from build123d import *

# Parameters (mm, degrees)
CROQUIS1_W              = 36
CROQUIS1_H              = 25
SALIENTE_EXTRUIR1_DEPTH = 25
CROQUIS2_W              = 31
CROQUIS2_H              = 25
CORTAR_EXTRUIR1_DEPTH   = 22
CROQUIS3_R              = 2.15
CORTAR_EXTRUIR2_DEPTH   = 37
CROQUIS3_3_R            = 2.65
CROQUIS3_3_R_2          = 2.15
CORTAR_EXTRUIR3_DEPTH   = 1.015
CROQUIS4_R              = 2.65
CROQUIS4_R_2            = 2.15
CORTAR_EXTRUIR4_DEPTH   = 1.015
CROQUIS5_W              = 31
CROQUIS5_H              = 25
SALIENTE_EXTRUIR2_DEPTH = 22
CROQUIS6_W              = 25.17
CROQUIS6_H              = 25
CORTAR_EXTRUIR5_DEPTH   = 22
CROQUIS8_R              = 2.15
CORTAR_EXTRUIR6_DEPTH   = 34.5
CROQUIS8_3_R            = 2.65
CROQUIS8_3_R_2          = 2.15
CORTAR_EXTRUIR7_DEPTH   = 1.015
CROQUIS10_R             = 2.65
CROQUIS10_R_2           = 2.15
CORTAR_EXTRUIR8_DEPTH   = 1.015
REDONDEO2_R             = 10
REDONDEO3_R             = 1
REDONDEO4_R             = 1
REDONDEO5_R             = 1


with BuildPart() as part:
    # Croquis1 → Saliente-Extruir1 (new body)
    with BuildSketch(Plane.XY):
        with Locations((18, 12.5)):
            Rectangle(CROQUIS1_W, CROQUIS1_H)
    extrude(amount=SALIENTE_EXTRUIR1_DEPTH)

    # Croquis2 → Cortar-Extruir1 (cut)
    with BuildSketch(Plane.XY.offset(25)):
        with Locations((18, 12.5)):
            Rectangle(CROQUIS2_W, CROQUIS2_H)
    extrude(amount=-CORTAR_EXTRUIR1_DEPTH, mode=Mode.SUBTRACT)

    # Croquis3 → Cortar-Extruir2 (cut, through all)
    with BuildSketch(Plane(origin=(36, 0, 0), x_dir=(0, 0, -1), z_dir=(1, 0, 0))):
        with Locations((-15.615366346, 18.5)):
            Circle(CROQUIS3_R)
        with Locations((-9.615366346, 12.5)):
            Circle(CROQUIS3_R)
        with Locations((-15.615366346, 12.5)):
            Circle(CROQUIS3_R)
        with Locations((-21.615366346, 12.5)):
            Circle(CROQUIS3_R)
        with Locations((-15.615366346, 6.5)):
            Circle(CROQUIS3_R)
    extrude(amount=-CORTAR_EXTRUIR2_DEPTH, mode=Mode.SUBTRACT)

    # Croquis3_3 → Cortar-Extruir3 (cut)
    with BuildSketch(Plane(origin=(36, 0, 0), x_dir=(0, 0, -1), z_dir=(1, 0, 0))):
        with Locations((-15.615366346, 18.5)):
            Circle(CROQUIS3_3_R)
        with Locations((-15.615366346, 18.5)):
            Circle(CROQUIS3_3_R_2, mode=Mode.SUBTRACT)
        with Locations((-9.615366346, 12.5)):
            Circle(CROQUIS3_3_R)
        with Locations((-9.615366346, 12.5)):
            Circle(CROQUIS3_3_R_2, mode=Mode.SUBTRACT)
        with Locations((-15.615366346, 12.5)):
            Circle(CROQUIS3_3_R)
        with Locations((-15.615366346, 12.5)):
            Circle(CROQUIS3_3_R_2, mode=Mode.SUBTRACT)
        with Locations((-21.615366346, 12.5)):
            Circle(CROQUIS3_3_R)
        with Locations((-21.615366346, 12.5)):
            Circle(CROQUIS3_3_R_2, mode=Mode.SUBTRACT)
        with Locations((-15.615366346, 6.5)):
            Circle(CROQUIS3_3_R)
        with Locations((-15.615366346, 6.5)):
            Circle(CROQUIS3_3_R_2, mode=Mode.SUBTRACT)
    extrude(amount=-CORTAR_EXTRUIR3_DEPTH, mode=Mode.SUBTRACT)

    # Croquis4 → Cortar-Extruir4 (cut)
    with BuildSketch(Plane.ZY):
        with Locations((15.615366346, 18.5)):
            Circle(CROQUIS4_R)
        with Locations((15.615366346, 18.5)):
            Circle(CROQUIS4_R_2, mode=Mode.SUBTRACT)
        with Locations((21.615366346, 12.5)):
            Circle(CROQUIS4_R)
        with Locations((21.615366346, 12.5)):
            Circle(CROQUIS4_R_2, mode=Mode.SUBTRACT)
        with Locations((15.615366346, 12.5)):
            Circle(CROQUIS4_R)
        with Locations((15.615366346, 12.5)):
            Circle(CROQUIS4_R_2, mode=Mode.SUBTRACT)
        with Locations((9.615366346, 12.5)):
            Circle(CROQUIS4_R)
        with Locations((9.615366346, 12.5)):
            Circle(CROQUIS4_R_2, mode=Mode.SUBTRACT)
        with Locations((15.615366346, 6.5)):
            Circle(CROQUIS4_R)
        with Locations((15.615366346, 6.5)):
            Circle(CROQUIS4_R_2, mode=Mode.SUBTRACT)
    extrude(amount=-CORTAR_EXTRUIR4_DEPTH, mode=Mode.SUBTRACT)

    # Croquis5 → Saliente-Extruir2 (add)
    with BuildSketch(Plane(origin=(0, 0, 0), x_dir=(-1, 0, 0), z_dir=(0, 0, -1))):
        with Locations((-18, 12.5)):
            Rectangle(CROQUIS5_W, CROQUIS5_H)
    extrude(amount=SALIENTE_EXTRUIR2_DEPTH)

    # Croquis6 → Cortar-Extruir5 (cut)
    with BuildSketch(Plane(origin=(0, 0, -22), x_dir=(-1, 0, 0), z_dir=(0, 0, -1))):
        with Locations((-18, 12.5)):
            Rectangle(CROQUIS6_W, CROQUIS6_H)
    extrude(amount=-CORTAR_EXTRUIR5_DEPTH, mode=Mode.SUBTRACT)

    # Croquis8 → Cortar-Extruir6 (cut, through all)
    with BuildSketch(Plane.ZY.offset(-2.5)):
        with Locations((-18, 21.75)):
            Circle(CROQUIS8_R)
        with Locations((-12, 21.75)):
            Circle(CROQUIS8_R)
        with Locations((-6, 21.75)):
            Circle(CROQUIS8_R)
        with Locations((-18, 3.25)):
            Circle(CROQUIS8_R)
        with Locations((-12, 3.25)):
            Circle(CROQUIS8_R)
        with Locations((-6, 3.25)):
            Circle(CROQUIS8_R)
    extrude(amount=-CORTAR_EXTRUIR6_DEPTH, mode=Mode.SUBTRACT)

    # Croquis8_3 → Cortar-Extruir7 (cut)
    with BuildSketch(Plane.ZY.offset(-2.5)):
        with Locations((-18, 21.75)):
            Circle(CROQUIS8_3_R)
        with Locations((-18, 21.75)):
            Circle(CROQUIS8_3_R_2, mode=Mode.SUBTRACT)
        with Locations((-6, 21.75)):
            Circle(CROQUIS8_3_R)
        with Locations((-6, 21.75)):
            Circle(CROQUIS8_3_R_2, mode=Mode.SUBTRACT)
        with Locations((-18, 3.25)):
            Circle(CROQUIS8_3_R)
        with Locations((-18, 3.25)):
            Circle(CROQUIS8_3_R_2, mode=Mode.SUBTRACT)
        with Locations((-6, 3.25)):
            Circle(CROQUIS8_3_R)
        with Locations((-6, 3.25)):
            Circle(CROQUIS8_3_R_2, mode=Mode.SUBTRACT)
        with Locations((-12, 21.75)):
            Circle(CROQUIS8_3_R)
        with Locations((-12, 21.75)):
            Circle(CROQUIS8_3_R_2, mode=Mode.SUBTRACT)
        with Locations((-12, 3.25)):
            Circle(CROQUIS8_3_R)
        with Locations((-12, 3.25)):
            Circle(CROQUIS8_3_R_2, mode=Mode.SUBTRACT)
    extrude(amount=-CORTAR_EXTRUIR7_DEPTH, mode=Mode.SUBTRACT)

    # Croquis10 → Cortar-Extruir8 (cut)
    with BuildSketch(Plane(origin=(33.5, 0, 0), x_dir=(0, 0, -1), z_dir=(1, 0, 0))):
        with Locations((6, 21.75)):
            Circle(CROQUIS10_R)
        with Locations((6, 21.75)):
            Circle(CROQUIS10_R_2, mode=Mode.SUBTRACT)
        with Locations((12, 21.75)):
            Circle(CROQUIS10_R)
        with Locations((12, 21.75)):
            Circle(CROQUIS10_R_2, mode=Mode.SUBTRACT)
        with Locations((18, 21.75)):
            Circle(CROQUIS10_R)
        with Locations((18, 21.75)):
            Circle(CROQUIS10_R_2, mode=Mode.SUBTRACT)
        with Locations((6, 3.25)):
            Circle(CROQUIS10_R)
        with Locations((6, 3.25)):
            Circle(CROQUIS10_R_2, mode=Mode.SUBTRACT)
        with Locations((12, 3.25)):
            Circle(CROQUIS10_R)
        with Locations((12, 3.25)):
            Circle(CROQUIS10_R_2, mode=Mode.SUBTRACT)
        with Locations((18, 3.25)):
            Circle(CROQUIS10_R)
        with Locations((18, 3.25)):
            Circle(CROQUIS10_R_2, mode=Mode.SUBTRACT)
    extrude(amount=-CORTAR_EXTRUIR8_DEPTH, mode=Mode.SUBTRACT)

    # Redondeo2
    redondeo2_edges = [part.edges().sort_by_distance(p)[0] for p in [
        (34.75, 25, 25),
        (34.75, 0, 25),
        (1.25, 25, 25),
        (1.25, 0, 25),
    ]]
    fillet(redondeo2_edges, radius=REDONDEO2_R)

    # Redondeo3
    redondeo3_edges = [part.edges().sort_by_distance(p)[0] for p in [
        (33.5, 12.5, 3),
    ]]
    fillet(redondeo3_edges, radius=REDONDEO3_R)

    # Redondeo4
    redondeo4_edges = [part.edges().sort_by_distance(p)[0] for p in [
        (2.5, 12.5, 3),
    ]]
    fillet(redondeo4_edges, radius=REDONDEO4_R)

    # Redondeo5
    redondeo5_edges = [part.edges().sort_by_distance(p)[0] for p in [
        (2.5, 12.5, 25),
        (2.5, 22.071067812, 22.071067812),
        (2.5, 2.928932188, 22.071067812),
        (33.5, 12.5, 25),
        (33.5, 22.071067812, 22.071067812),
        (33.5, 2.928932188, 22.071067812),
        (18, 25, 3),
        (33.5, 0, 9.5),
        (33.5, 25, 9.5),
        (33.207106781, 25, 3.292893219),
        (33.207106781, 0, 3.292893219),
        (18, 0, 3),
        (2.5, 0, 9.5),
        (2.5, 25, 9.5),
        (2.792893219, 0, 3.292893219),
        (2.792893219, 25, 3.292893219),
    ]]
    fillet(redondeo5_edges, radius=REDONDEO5_R)


solid = part.part
The listing builds one solid part. Answer for the finished solid, in the listing's coordinates (mm). A direction names the side the tool comes from. Coordinates: 2 decimals unless noted, no trailing zeros. Loops run counter-clockwise (first coordinate to the right, second up) from the corner with the lowest first, then second, coordinate; pieces in that order, holes last. Notation, with made-up numbers: (13.5, 31) -> (72.5, 31) arc R26 ccw to (72.5, 48) -> close; hole circle Ø8 at (43, 48). An arc over 180 degrees is marked (long way). Write item = value, one per line. Start each with the question number.
1) A tool of negligible diameter and unlimited length cuts with its end or side. For faces 4 (the face through (35.5, 10.89, 17.72)), 5 (the face through (3.515, 24, -13)), 6 (the face through (1, 13, 0)), 7 (the face through (0.76, 3.01, 22.15)), 8 (the face through (17.797, 0.301, 2.715)), from which of +Z, -Z, +X, -X, +Y, -Y can it reach the whole face along a straight path? Write none if from no direction.
2) A cutting plane is placed at A-A (y = 12.5). Count the separate pieces of the cut face and the enclosed holes in it, then the cut area to 3 significant figures.
3) A cutting plane is placed at B-B (x = 21.5). Give the vertices of the cut face in (y, z).
4) The mould has two halves that part along X. Classify faces 1 (the face through (18, 13, 3)), 2 (the face through (33, 19.16, -5.43)), 3 (the face through (36, 9.5, 9.5)): released by +X, released by -X, zero draft, split by the parting line, or undercut.
5) Straight lines are drawn through the part: line 1 (Y direction, x = 32.95, z = -6); line 2 (Y direction, x = 31.6, z = -12); line 3 (X direction, y = 5.5, z = -10) (3 decimals). For each, find the intervals that lie inside material, in ascending order. Write a range as from..to.
6) Given pin 1 Ø3 at (x, y) = (20.5, 14.5) entering from +Z; pin 2 Ø3.5 at (y, z) = (18.5, 15.62) entering from +X; pin 3 Ø4 at (y, z) = (13.5, 20.5) entering from -X; pin 4 Ø10 at (x, z) = (6.5, 16.5) entering from +Y, each flat-ended and moving along its own axis, determine where each tip first touches the part or whether it passes through.
Responses:
q1.face_4 = +X
q1.face_5 = -X
q1.face_6 = -Z, -X, +Y, -Y
q1.face_7 = +Z, +X, -X, -Y
q1.face_8 = +Z, -Y
q2.separate_pieces = 7
q2.enclosed_holes = 0
q2.area = 276 mm²
q3.outline = (0, 0) -> (25, 0) -> (25, 2) arc R1 ccw to (24, 3) -> (1, 3) arc R1 ccw to (0, 2) -> close
q4.face_1 = undercut
q4.face_2 = zero draft
q4.face_3 = released by +X
q5.line_1 = 0..0.6, 5.9..19.1, 24.4..25
q5.line_2 = 0..1.1, 5.4..19.6, 23.9..25
q5.line_3 = 2.5..5.415, 30.585..33.5
q6.pin_1 = 3
q6.pin_2 = through
q6.pin_3 = 0
q6.pin_4 = 24.98
